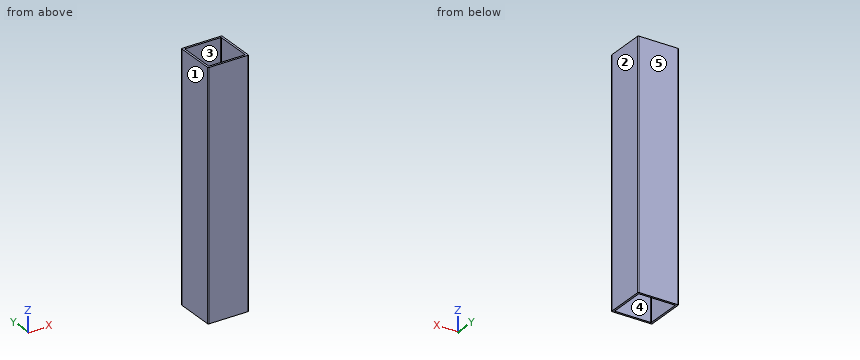
from build123d import *

# Parameters (mm, degrees)
SKETCH1_W           = 25.4
SKETCH1_H           = 25.4
SKETCH1_W_2         = 22.9108
SKETCH1_H_2         = 22.9108
BOSS_EXTRUDE1_DEPTH = 152.4
FILLET1_R           = 0.4064
FILLET2_R           = 0.4064


with BuildPart() as part:
    # Sketch1 → Boss-Extrude1 (new body)
    with BuildSketch(Plane.XY):
        with Locations((12.7, 12.7)):
            Rectangle(SKETCH1_W, SKETCH1_H)
        with Locations((12.7, 12.7)):
            Rectangle(SKETCH1_W_2, SKETCH1_H_2, mode=Mode.SUBTRACT)
    extrude(amount=-BOSS_EXTRUDE1_DEPTH)

    # Fillet1
    fillet1_edges = [part.edges().sort_by_distance(p)[0] for p in [
        (0, 25.4, -76.2),
        (25.4, 25.4, -76.2),
        (25.4, 0, -76.2),
        (0, 0, -76.2),
    ]]
    fillet(fillet1_edges, radius=FILLET1_R)

    # Fillet2
    fillet2_edges = [part.edges().sort_by_distance(p)[0] for p in [
        (1.2446, 1.2446, -76.2),
        (1.2446, 24.1554, -76.2),
        (24.1554, 24.1554, -76.2),
        (24.1554, 1.2446, -76.2),
    ]]
    fillet(fillet2_edges, radius=FILLET2_R)


solid = part.part
Source: CAD feature listing. Evaluate the final solid. Frame: model axes, mm. Face numbers are marked on the shaded views. A direction names the side the tool comes from. Round coordinates to 2 decimals unless told otherwise and drop trailing zeros. Order: outer loops, then holes, each group sorted by start corner. A loop starts at its lowest first (then second) coordinate and runs counter-clockwise, first axis right, second up. Notation, with made-up numbers: (-38.5, 82.5) - (-4.5, 82.5) arc R28 cw to (-4.5, 107.5) - close; hole circle Ø3 at (-15, -25). An arc over 180 degrees is marked (long way). Use a Markdown table: item, result. Add a question column.
1. Set-up query: the marked faces 4 and 5. Return all of +Z, -Z, +X, -X, +Y, -Y with unobstructed straight access to the full face (end or side cutting, diameter ignored); none if empty.
2. Line query: probe 1 along X at (y, z) = (18.5, -16). Output: solid intervals per line, ascending.
3. Section query C-C (z = -139). Return the cut outline in (x, y).
4. Section query A-A (x = 7.75). Return the cut outline in (y, z).
5. Mould query, pull axis X, two halves, no side actions, for the marked faces 1, 2 and 3. Classes: +X half, -X half, draft (parallel to the pull), parting line (faces both ways), or undercut.
Derived:
| question | item | result |
|---|---|---|
| 1 | face 4 | +Z, -Z |
| 1 | face 5 | +Z, -Z, +X, -X, +Y |
| 2 | probe 1 | 0 to 1.24, 24.16 to 25.4 |
| 3 | outline | (0, 0.41) arc R0.41 ccw to (0.41, 0) - (24.99, 0) arc R0.41 ccw to (25.4, 0.41) - (25.4, 24.99) arc R0.41 ccw to (24.99, 25.4) - (0.41, 25.4) arc R0.41 ccw to (0, 24.99) - close; hole (1.24, 1.65) arc R0.41 ccw to (1.65, 1.24) - (23.75, 1.24) arc R0.41 ccw to (24.16, 1.65) - (24.16, 23.75) arc R0.41 ccw to (23.75, 24.16) - (1.65, 24.16) arc R0.41 ccw to (1.24, 23.75) - close |
| 4 | outline | (0, -152.4) - (1.24, -152.4) - (1.24, 0) - (0, 0) - close; (24.16, -152.4) - (25.4, -152.4) - (25.4, 0) - (24.16, 0) - close |
| 5 | face 1 | -X half |
| 5 | face 2 | +X half |
| 5 | face 3 | undercut |
